The drawing under review shows one solid part. Ordinate dimensions are in mm from its lowest x, y, z. A direction names the side the tool comes from. Coordinates: 2 decimals unless noted, no trailing zeros. Write each loop counter-clockwise with the first axis right and the second up, starting at its lowest first coordinate (ties: lowest second). Pieces come first, ordered by that corner, then holes.
1) Add section C-C, the plane z = 85. State the section outline as (x, y) points, then the cut area to 3 significant figures.
2) Mouldability with a two-part tool opening along Z and no side actions: class the marked faces 4, 5, 6 and 7 as released by +Z, released by -Z, zero draft, split by the parting line, or undercut.
3) Add section A-A, the plane y = 25.5. State the section outline as (x, z) points, then the cut area to 3 significant figures.
4) Machinability: for the marked faces 1, 2 and 3, which of the approach directions +Z, -Z, +X, -X, +Y, -Y give a long, thin tool a straight path to every point of the face, cutting with its end or side? Answer none if there is none.
5) For line 1 (Z direction, x = 202.5, y = 46.2); line 2 (X direction, y = 18.5, z = 107); line 3 (X direction, y = 46.5, z = 130.5), list the stretches that pass through material, from the lowest coordinate up.
6) Add section B-B, the plane x = 190. State the section outline as (y, z) points, then the cut area to 4 significant figures.
7) For P1, Ø2, axis at x = 99.5, y = 43, coming from the -Z side; P2, Ø5.5, axis at x = 121.5, z = 16.5, coming from the -Y side; P3, Ø1, axis at x = 32, z = 63, coming from the +Y side, all flat-tipped, find the tip position at first contact; note any pin that passes through.
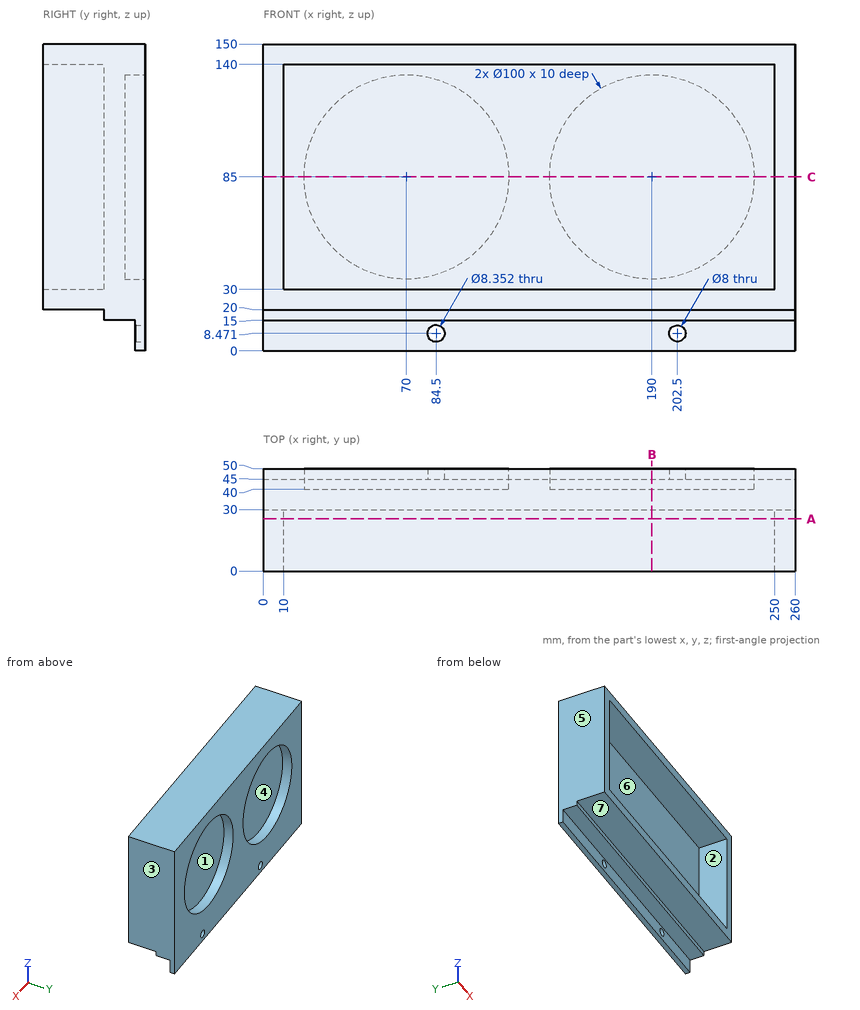
Geometry results:
1. outline: (0, 0) - (10, 0) - (10, 30) - (250, 30) - (250, 0) - (260, 0) - (260, 50) - (240, 50) - (240, 40) - (140, 40) - (140, 50) - (120, 50) - (120, 40) - (20, 40) - (20, 50) - (0, 50) - close
1. area: 3,800 mm2
2. face 4: undercut
2. face 5: zero draft
2. face 6: undercut
2. face 7: released by -Z
3. outline: (0, 20) - (260, 20) - (260, 150) - (0, 150) - close; hole (10, 30) - (250, 30) - (250, 140) - (10, 140) - close
3. area: 7,400 mm2
4. face 1: +Y
4. face 2: -Y
4. face 3: +Z, -Z, +X, +Y, -Y
5. line 1: z = 0 to 4.47, 12.47 to 36.59, 133.41 to 150
5. line 2: x = 0 to 10, 250 to 260
5. line 3: x = 0 to 49.27, 90.73 to 169.27, 210.73 to 260
6. outline: (0, 20) - (30, 20) - (30, 15) - (45, 15) - (45, 0) - (50, 0) - (50, 35) - (40, 35) - (40, 135) - (50, 135) - (50, 150) - (0, 150) - (0, 140) - (30, 140) - (30, 30) - (0, 30) - close
6. area: 2,375 mm2
7. P1: stops at z = 15
7. P2: stops at y = 30
7. P3: stops at y = 40
